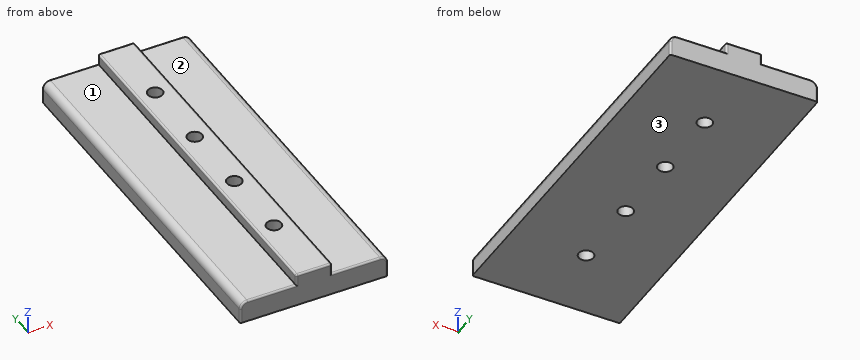
```python
from build123d import *

# Parameters (mm, degrees)
F1_DEPTH = 100
F2_R     = 2
F3_DEPTH = 9
F4_R     = 0.5


with BuildPart() as f1:
    # F0 (on Front) → F1 (new body)
    with BuildSketch(Plane.XZ):
        with BuildLine():
            Line((-13.1858391894, 0), (26.8141608106, 0))
            Line((26.8141608106, 0), (26.8141608106, 4))
            ThreePointArc((26.8141608106, 4), (26.228374373, 5.4142135624), (24.8141608106, 6))
            Line((24.8141608106, 6), (11.6891608106, 6))
            Line((11.6891608106, 6), (11.6891608106, 8.5))
            ThreePointArc((11.6891608106, 8.5), (11.5427142012, 8.8535533906), (11.1891608106, 9))
            Line((11.1891608106, 9), (2.4391608106, 9))
            ThreePointArc((2.4391608106, 9), (2.08560742, 8.8535533906), (1.9391608106, 8.5))
            Line((1.9391608106, 8.5), (1.9391608106, 6))
            Line((1.9391608106, 6), (-11.1858391894, 6))
            ThreePointArc((-11.1858391894, 6), (-12.6000527518, 5.4142135624), (-13.1858391894, 4))
            Line((-13.1858391894, 4), (-13.1858391894, 0))
        make_face()
    extrude(amount=F1_DEPTH)

    # F2 (on face) → F3 (cut, through all)
    with BuildSketch(Plane.XY.offset(9)):
        with Locations((6.6891608106, -80)):
            Circle(F2_R)
        with Locations((6.6891608106, -60)):
            Circle(F2_R)
        with Locations((6.6891608106, -40)):
            Circle(F2_R)
        with Locations((6.6891608106, -20)):
            Circle(F2_R)
    extrude(amount=-F3_DEPTH, mode=Mode.SUBTRACT)

    # F4
    f4_edges = [f1.edges().sort_by_distance(p)[0] for p in [
        (18.251661, -100, 6),
        (6.814161, -100, 9),
        (-4.623339, -100, 6),
        (11.689161, -100, 7.25),
        (11.542714, -100, 8.853553),
        (2.085607, -100, 8.853553),
        (1.939161, -100, 7.25),
        (-13.185839, -100, 2),
        (-12.600053, -100, 5.414214),
        (26.228374, -100, 5.414214),
        (26.814161, -100, 2),
        (-13.185839, 0, 2),
        (-12.600053, 0, 5.414214),
        (1.939161, 0, 7.25),
        (2.085607, 0, 8.853553),
        (6.814161, 0, 9),
        (18.251661, 0, 6),
        (26.228374, 0, 5.414214),
    ]]
    fillet(f4_edges, radius=F4_R)


solid = f1.part
```
The model under review builds one solid part; all positions refer to its coordinate system, in mm. Face numbers are marked on the shaded views. A direction names the side the tool comes from. Coordinates: 2 decimals unless noted, no trailing zeros. Write each loop counter-clockwise with the first axis right and the second up, starting at its lowest first coordinate (ties: lowest second). Pieces come first, ordered by that corner, then holes. Notation, with made-up numbers: (33.5, -35) - (55.5, -35) arc R21 cw to (55.5, -22) - close; hole circle Ø8 at (85.5, 19.25). An arc over 180 degrees is marked (long way). Write item = value, one per line.
(1) Consider section A-A, the plane y = -40. Give the boundary of the cut face in (x, z), then the cut area to 3 significant figures.
Result sheet:
outline = (-13.19, 0) - (4.69, 0) - (4.69, 9) - (2.44, 9) arc R0.5 ccw to (1.94, 8.5) - (1.94, 6) - (-11.19, 6) arc R2 ccw to (-13.19, 4) - close; (8.69, 0) - (26.81, 0) - (26.81, 4) arc R2 ccw to (24.81, 6) - (11.69, 6) - (11.69, 8.5) arc R0.5 ccw to (11.19, 9) - (8.69, 9) - close
area = 231 mm^2
(2) Consider section B-B, the plane y = -50. Give the boundary of the cut face in (x, z), then the cut area to 3 significant figures.
Result sheet:
outline = (-13.19, 0) - (26.81, 0) - (26.81, 4) arc R2 ccw to (24.81, 6) - (11.69, 6) - (11.69, 8.5) arc R0.5 ccw to (11.19, 9) - (2.44, 9) arc R0.5 ccw to (1.94, 8.5) - (1.94, 6) - (-11.19, 6) arc R2 ccw to (-13.19, 4) - close
area = 267 mm^2
(3) Consider section C-C, the plane x = 7. Give the boundary of the cut face in (y, z), then the cut area to 3 significant figures.
Result sheet:
outline = (-100, 0) - (-81.98, 0) - (-81.98, 9) - (-99.5, 9) arc R0.5 ccw to (-100, 8.5) - close; (-78.02, 0) - (-61.98, 0) - (-61.98, 9) - (-78.02, 9) - close; (-58.02, 0) - (-41.98, 0) - (-41.98, 9) - (-58.02, 9) - close; (-38.02, 0) - (-21.98, 0) - (-21.98, 9) - (-38.02, 9) - close; (-18.02, 0) - (0, 0) - (0, 8.5) arc R0.5 ccw to (-0.5, 9) - (-18.02, 9) - close
area = 758 mm^2
(4) For P1, Ø6, axis at x = -0.5, y = -72, coming from the +Z side; P2, Ø4, axis at x = 18.5, y = -55.5, coming from the +Z side; P3, Ø3, axis at y = -37, z = 7, coming from the -X side; P4, Ø1.2, axis at y = -52, z = 7, coming from the +X side, all flat-tipped, find the tip position at first contact; note any pin that passes through.
Result sheet:
P1 = 9
P2 = 6
P3 = -12.51
P4 = 11.69
(5) Consider section D-D, the plane x = 13.5. Give the boundary of the cut face in (y, z), then the cut area to 3 significant figures.
Result sheet:
outline = (-100, 0) - (0, 0) - (0, 5.5) arc R0.5 ccw to (-0.5, 6) - (-99.5, 6) arc R0.5 ccw to (-100, 5.5) - close
area = 600 mm^2
(6) Machinability: for the marked faces 1, 2 and 3, which of the approach directions +Z, -Z, +X, -X, +Y, -Y give a long, thin tool a straight path to every point of the face, cutting with its end or side? Answer none if there is none.
Result sheet:
face_1 = +Z, -X, +Y, -Y
face_2 = +Z, +X, +Y, -Y
face_3 = -Z, +X, -X, +Y, -Y
(7) For line 1 (Z direction, x = 20.5, y = -23); line 2 (X direction, y = -75, z = 6.25); line 3 (X direction, y = -41.5, z = 2.75), list the stretches that pass through material, from the lowest coordinate up. Write a range as [from, to].
Result sheet:
line_1 = [0, 6]
line_2 = [1.94, 11.69]
line_3 = [-13.19, 5.37], [8.01, 26.81]
